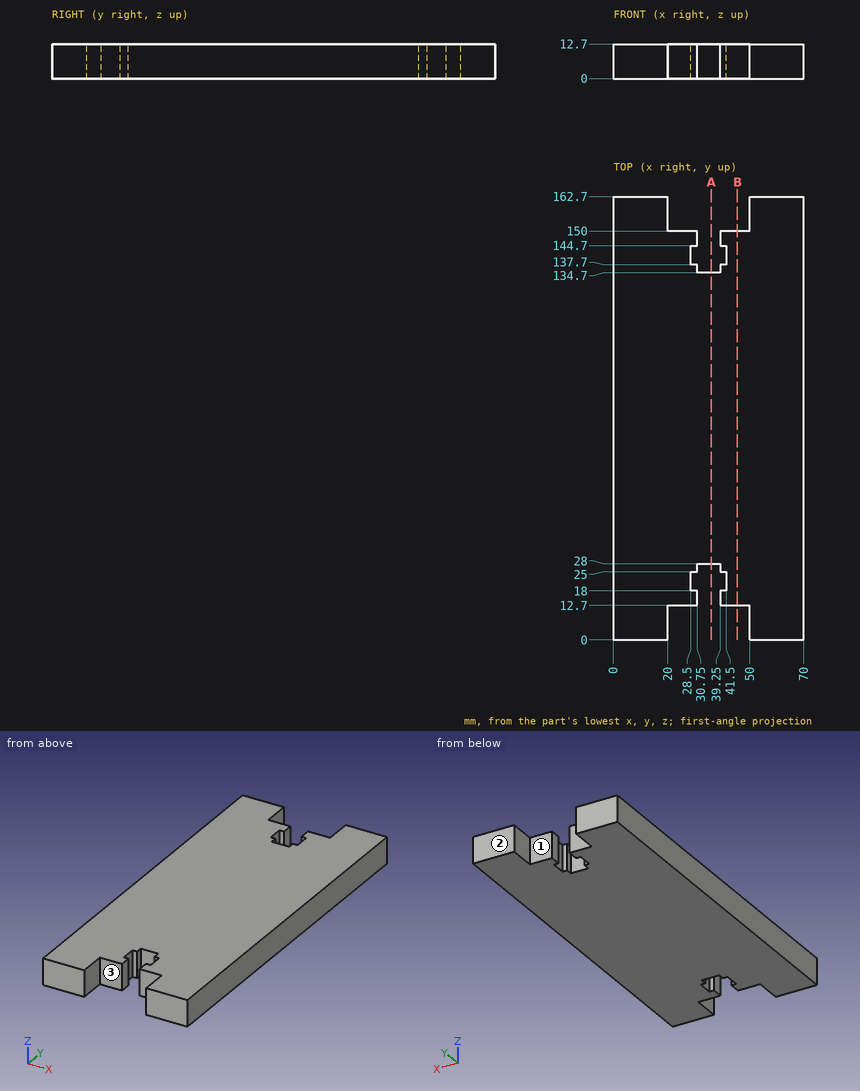
Design review of the part shown in the three views and the two pictorial views. Dimensions are in mm from the part's minimum x, y and z. A direction names the side the tool comes from. Give positions to 0.01 mm unless a question says otherwise; leave off trailing zeros. Order: outer loops, then holes, each group sorted by start corner. A loop starts at its lowest first (then second) coordinate and runs counter-clockwise, first axis right, second up. Notation, with made-up numbers: M -35,-34.5 L 8,-34.5 A21 ccw 8,-29.5 Z; hole C 5.25,-29.75 d7. An arc over 180 degrees is marked long. Answer in a Markdown table with one row per item. Add a question column.
(1) For the marked faces 1, 2 and 3, list the 3-axis set-ups (+Z, -Z, +X, -X, +Y, -Y) from which the entire face can be reached by the end or side of a thin tool; tool diameter is ignored.
(2) For pin 1 (2 mm diameter, centred on x = 24, z = 4, fed in from +Y); pin 2 (1.1 mm diameter, centred on x = 29.5, z = 5.5, fed in from -Y); pin 3 (2 mm diameter, centred on x = 34.5, z = 3.5, fed in from +Y), all flat-tipped, find the tip position at first contact; note any pin that passes through.
(3) Consider section B-B on x = 45.5. State the section outline as (y, z) points, and give its area (3 significant figures).
(4) Wall thickness on probe 1 along Y at (x, z) = (41, 1); probe 2 along X at (y, z) = (142, 6.25); probe 3 along X at (y, z) = (15, 1.75): over which ranges is each line inside the solid? List them lowest first. Write a range as [from, to].
(5) Consider section A-A on x = 36. State the section outline as (y, z) points.
Evaluation:
| question | item | result |
|---|---|---|
| 1 | face 1 | +Z, -Z, +Y |
| 1 | face 2 | +Z, -Z, +X, -X, +Y |
| 1 | face 3 | +Z, -Z, -Y |
| 2 | pin 1 | stops at y = 150 |
| 2 | pin 2 | stops at y = 12.7 |
| 2 | pin 3 | stops at y = 134.7 |
| 3 | outline | M 12.7,0 L 150,0 L 150,12.7 L 12.7,12.7 Z |
| 3 | area | 1,740 mm^2 |
| 4 | probe 1 | y = [12.7, 18], [25, 137.7], [144.7, 150] |
| 4 | probe 2 | x = [0, 28.5], [41.5, 70] |
| 4 | probe 3 | x = [0, 30.75], [39.25, 70] |
| 5 | outline | M 28,0 L 134.7,0 L 134.7,12.7 L 28,12.7 Z |
